Source: CAD feature listing. Evaluate the final solid. Frame: model axes, mm. A direction names the side the tool comes from. Round coordinates to 2 decimals unless told otherwise and drop trailing zeros. Write each loop counter-clockwise with the first axis right and the second up, starting at its lowest first coordinate (ties: lowest second). Pieces come first, ordered by that corner, then holes.
Autodesk Inventor part; units mm, degrees
ref_plane "YZ Plane" through (0, 0, 0) normal (1, 0, 0) x (0, 1, 0)
ref_plane "XZ Plane" through (0, 0, 0) normal (0, 1, 0) x (-1, 0, 0)
ref_plane "XY Plane" through (0, 0, 0) normal (0, 0, 1) x (1, 0, 0)
sketch "Esboço1" plane through (0, 0, 0) normal (0, 1, 0) x (-1, 0, 0)
  line L0 (75, 90) -> (-75, 90)
  line L1 (-75, 90) -> (-75, -90)
  line L2 (-75, -90) -> (75, -90)
  line L3 (75, -90) -> (75, 90)
  line L4 (75, 90) -> (-75, -90) construction
  line L5 (-75, 90) -> (75, -90) construction
  line L6 (50.5, 80) -> (-50.5, 80) construction
  line L7 (-50.5, 80) -> (-50.5, -8) construction
  line L8 (-50.5, -8) -> (50.5, -8) construction
  line L9 (50.5, -8) -> (50.5, 80) construction
  line L10 (50.5, 80) -> (-50.5, -8) construction
  line L11 (-50.5, 80) -> (50.5, -8) construction
  line L12 (35, -30) -> (-35, -30) construction
  line L13 (-35, -30) -> (-35, -80) construction
  line L14 (-35, -80) -> (35, -80) construction
  line L15 (35, -80) -> (35, -30) construction
  line L16 (35, -30) -> (-35, -80) construction
  line L17 (-35, -30) -> (35, -80) construction
  line L18 (0, 90) -> (0, -90) construction
  line L19 (80, 95) -> (-80, 95)
  line L20 (-80, 95) -> (-80, -95)
  line L21 (-80, -95) -> (80, -95)
  line L22 (80, -95) -> (80, 95)
  point P0 (0, 0)
  point P1 (0, 36)
  point P2 (0, -55)
  dimension "d0" = 150
  dimension "d1" = 180
  dimension "d2" = 101
  dimension "d3" = 88
  dimension "d4" = 70
  dimension "d5" = 50
  dimension "d6" = 10
  dimension "d7" = 10
  dimension "d8" = 5
extrude "Extrusão1" add sketch "Esboço1" along normal blind 50
extrude "Extrusion2" add sketch "Esboço1" along normal blind 4 contours L3 L2 L1 L0
sketch "SaidaCarga" plane through (80, 0, 95) normal (1, 0, 0) x (0, 0, -1)
  line L0 (0, 50) -> (190, 50)
  line L1 (0, 50) -> (190, 0) construction
  circle A0 centre (95, 25) radius 5
  circle A1 centre (95, 25) radius 7
  point P0 (95, 0)
  dimension "d13" = 10
  dimension "d14" = 2
sketch "Sketch3" plane through (0, 4, 0) normal (0, 1, 0) x (1, 0, 0)
  line L0 (-50.5, -80) -> (50.5, -80) construction
  line L1 (50.5, -80) -> (50.5, 8) construction
  line L2 (-50.5, 8) -> (-50.5, -80) construction
  line L3 (50.5, 8) -> (-50.5, 8) construction
  line L4 (-35, 30) -> (35, 30) construction
  line L5 (35, 30) -> (35, 80) construction
  line L6 (35, 80) -> (-35, 80) construction
  line L7 (-35, 80) -> (-35, 30) construction
  circle A0 centre (60, 55) radius 5
  circle A1 centre (60, 55) radius 7
  line L8 (75, 90) -> (75, -90)
  line L9 (-75, 90) -> (75, 90)
  line L10 (-35, 30) -> (35, 30)
  line L11 (35, 30) -> (35, 80)
  line L12 (35, 80) -> (-35, 80)
  line L13 (-35, 80) -> (-35, 30)
  circle A2 centre (-32.8, 32.2) radius 1.1
  line L14 (-35, 55) -> (35, 55) construction
  circle A3 centre (-32.8, 77.8) radius 1.1
  line L15 (0, 30) -> (0, 80) construction
  circle A4 centre (32.8, 32.2) radius 1.1
  circle A5 centre (32.8, 77.8) radius 1.1
  line L16 (-30.6, 34.4) -> (-35, 30) construction
  line L17 (-35, 34.4) -> (-30.6, 30) construction
  line L18 (-30.6, 80) -> (-30.6, 30)
  line L19 (30.6, 80) -> (30.6, 30)
  line L20 (-50.5, -75) -> (50.5, -75)
  line L21 (-40.5, 8) -> (-40.5, -80)
  line L22 (50.5, 3) -> (-50.5, 3)
  line L23 (40.5, -80) -> (40.5, 8)
  line L24 (-50.5, 8) -> (50.5, 8)
  line L25 (50.5, 8) -> (50.5, -80)
  line L26 (50.5, -80) -> (-50.5, -80)
  line L27 (-50.5, -80) -> (-50.5, 8)
  point P0 (0, 0)
  point P1 (30.6, 30)
  point P2 (40.5, 8)
  point P3 (-40.5, 3)
  point P4 (40.5, 3)
  point P5 (40.5, -75)
  point P6 (-40.5, -75)
  dimension "d15" = 10
  dimension "d16" = 2
  dimension "d17" = 15
  dimension "d18" = 35
  dimension "d29" = 2.2
  dimension "d30" = 2.2
  dimension "d31" = 2.2
  dimension "d32" = 4.4
  dimension "d35" = 5
  dimension "d36" = 10
  dimension "d37" = 5
  dimension "d38" = 10
extrude "Extrusion3" cut sketch "Sketch3" against normal blind 4 contours A0
extrude "Extrusion4" add sketch "Sketch3" along normal blind 2 contours A1
extrude "Extrusion5" cut sketch "SaidaCarga" against normal blind 5 contours A0
extrude "Extrusion6" add sketch "SaidaCarga" along normal blind 2 and the other way blind 7
extrude "Extrusion7" add sketch "Sketch3" along normal blind 5 contours L13 L12 L18 L10 | L19 L12 L11 L10 | A2 | A3 | A4 | A5
extrude "Extrusion8" add sketch "Sketch3" along normal blind 30 contours L20 L23 L26 L21 | L21 L24 L23 L22
fillet "Fillet1" radius 5 4 edges at (0, 4, -90) (-75, 4, 0) (0, 4, 90) (75, 4, 0)
fillet "Fillet2" radius 3 19 edges at (0, 4, -3) (40.5, 4, -5.5) (0, 4, -8) (-40.5, 4, -5.5) (0, 4, 75) (-40.5, 4, 77.5) (0, 4, 80) (40.5, 4, 77.5) (35, 4, -55) (30.6, 4, -55) (32.8, 4, -30) (32.8, 4, -80) (-30.6, 4, -55) (-32.8, 4, -30) (-35, 4, -55) (-32.8, 4, -80) (80, 25, 7) (75, 25, 7) (53, 4, -55)
properties part number "CaseBitDog"
1) Contact query for flat-ended pins moving along their axis: P1, Ø15, axis at y = 33, z = 7, coming from the +X side; P2, Ø1, axis at y = 8.5, z = -45.5, coming from the +X side; P3, Ø2, axis at x = -1, z = 30, coming from the +Y side; P4, Ø1.3, axis at x = -32, z = -65.5, coming from the +Y side. Output: stop coordinate, or through.
Taken from the geometry:
P1: stops at x = 82
P2: stops at x = 80
P3: stops at y = 4
P4: stops at y = 9
2) Material intervals for line 1 (Z direction, x = 60, y = 3); line 2 (Z direction, x = 13, y = 16); line 3 (Z direction, x = -24, y = 46), sorted ascending.
Taken from the geometry:
line 1: z = -95 to -60, -50 to 95
line 2: z = -95 to -90, -8 to -3, 75 to 80, 90 to 95
line 3: z = -95 to -90, 90 to 95
3) Pull-direction query (X, two-part tool) for faces 1 (the face through (1, 0, 1)), 2 (the face through (-33, 9, -55)), 3 (the face through (82, 30, 2)); classes: released by +X, released by -X, zero draft, split by the parting line, or undercut.
Taken from the geometry:
face 1: zero draft
face 2: undercut
face 3: released by +X
4) Section query B-B on y = 25. Return the cut outline in (x, z), then the cut area to 3 significant figures.
Taken from the geometry:
outline: (-80, -95) - (80, -95) - (80, -9.83) arc R3 cw to (82, -7) - (82, -5) - (73, -5) - (73, -7) arc R3 cw to (75, -9.83) - (75, -90) - (-75, -90) - (-75, 90) - (75, 90) - (75, 9.83) arc R3 cw to (73, 7) - (73, 5) - (82, 5) - (82, 7) arc R3 cw to (80, 9.83) - (80, 95) - (-80, 95) - close; (-40.5, -8) - (40.5, -8) - (40.5, -3) - (-40.5, -3) - close; (-40.5, 75) - (40.5, 75) - (40.5, 80) - (-40.5, 80) - close
area: 4,180 mm2
5) Section query A-A on x = 60. Return the cut outline in (y, z).
Taken from the geometry:
outline: (0, -95) - (50, -95) - (50, -90) - (9, -90) arc R5 cw to (4, -85) - (4, -64.83) arc R3 cw to (6, -62) - (6, -60) - (0, -60) - close; (0, -50) - (6, -50) - (6, -48) arc R3 cw to (4, -45.17) - (4, 85) arc R5 cw to (9, 90) - (50, 90) - (50, 95) - (0, 95) - close
6) Reachability of faces 4 (the face through (77, 50, 0)), 5 (the face through (1, 20, -3)) from +Z, -Z, +X, -X, +Y, -Y: full face, straight path, thin tool, end or side. Return the list, or none.
Taken from the geometry:
face 4: +Z, -Z, +X, -X, +Y
face 5: +Y
7) Section query D-D on x = -17. Return the cut outline in (y, z), then the cut area to 3 significant figures.
Taken from the geometry:
outline: (0, -95) - (50, -95) - (50, -90) - (9, -90) arc R5 cw to (4, -85) - (4, -11) arc R3 cw to (7, -8) - (34, -8) - (34, -3) - (7, -3) arc R3 cw to (4, 0) - (4, 72) arc R3 cw to (7, 75) - (34, 75) - (34, 80) - (7, 80) arc R3 cw to (4, 83) - (4, 85) arc R5 cw to (9, 90) - (50, 90) - (50, 95) - (0, 95) - close
area: 1,540 mm2
